The model under review builds one solid part; all positions refer to its coordinate system, in mm. Face numbers are marked on the shaded views. A direction names the side the tool comes from. Coordinates: 2 decimals unless noted, no trailing zeros. Loops run counter-clockwise (first coordinate to the right, second up) from the corner with the lowest first, then second, coordinate; pieces in that order, holes last. Notation, with made-up numbers: M -29,0 L 5,0 A20 cw 5,39 Z; hole C 86.5,81.5 d3. An arc over 180 degrees is marked long. Use one line per item in the form item = value.
Autodesk Fusion 360 part; units mm, degrees
sketch "Sketch1" plane through (0, 0, 0) normal (0, 1, 0) x (1, 0, 0)
  line L0 (65, -5) -> (65, -14.5431)
  line L1 (14.2436, -31.1356) -> (24.2436, -31.1356)
  line L2 (24.2436, -101.1356) -> (14.2436, -101.1356)
  line L3 (14.2436, -101.1356) -> (14.2436, -31.1356)
  line L4 (24.2436, -31.1356) -> (74.2436, -31.1356)
  line L5 (74.2436, -31.1356) -> (74.2436, -41.1356)
  line L6 (74.2436, -41.1356) -> (24.2436, -41.1356)
  line L7 (24.2436, -41.1356) -> (24.2436, -101.1356)
  dimension "d5" = 10
  dimension "d6" = 70
  dimension "d7" = 50
  dimension "d8" = 10
extrude "Extrude1" add sketch "Sketch1" along normal blind 30
sketch "Sketch2" plane through (0, 0, 0) normal (0, 0, 1) x (1, 0, 0)
  circle A0 centre (36, 20) radius 2
  dimension "d11" = 4
extrude "Extrude2" cut sketch "Sketch2" along normal blind 72
pattern_linear "R-Pattern1" count 3 spacing 13 along (1, 0, 0) count 2 spacing 11 along (0, -1, 0) of "Extrude2"
sketch "Sketch3" plane through (0, 0, 0) normal (1, 0, 0) x (0, 0, -1)
  circle A0 centre (-58.7967, 22.3764) radius 2
  dimension "d18" = 4
extrude "Extrude3" cut sketch "Sketch3" along normal blind 50
pattern_linear "R-Pattern2" count 3 spacing 15 along (0, 0, 1) count 2 spacing 15 along (0, -1, 0) of "Extrude3"
fillet "Fillet1" radius 0.5 6 edges at (49.2436, 30, 41.1356) (74.2436, 15, 41.1356) (24.2436, 30, 71.1356) (24.2436, 15, 101.1356) (24.2436, 0, 71.1356) (49.2436, 0, 41.1356)
chamfer "Chamfer1" distance 1 angle 45 12 edges at (34.1353, 9.7232, 41.1356) (47.1353, 9.7232, 41.1356) (60.1353, 9.7232, 41.1356) (60.1353, 20.7232, 41.1356) (47.1353, 20.7232, 41.1356) (34.1353, 20.7232, 41.1356) (24.2436, 8.0997, 60.6613) (24.2436, 8.0997, 75.6613) (24.2436, 8.0997, 90.6613) (24.2436, 23.0997, 75.6613) (24.2436, 23.0997, 90.6613) (24.2436, 23.0997, 60.6613)
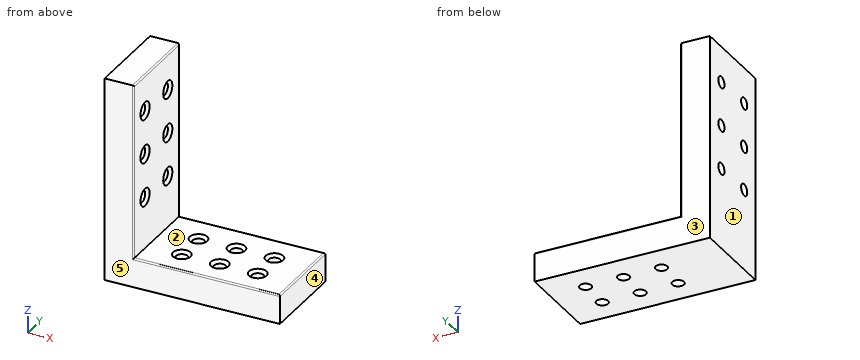
1. Add section A-A (x = 62). State the section outline as (y, z) points.
Response values:
outline = M 0,31.14 L 7,31.14 L 7,40.14 L 6,41.14 L 0.5,41.14 A0.5 ccw 0,40.64 Z; M 11,31.14 L 18,31.14 L 18,40.14 L 17,41.14 L 12,41.14 L 11,40.14 Z; M 22,31.14 L 30,31.14 L 30,40.64 A0.5 ccw 29.5,41.14 L 23,41.14 L 22,40.14 Z
2. Insertion check: P1, Ø1.5, axis at y = 20.5, z = 84, coming from the +X side; P2, Ø3, axis at x = 57, y = 7, coming from the +Z side; P3, Ø4.5, axis at x = 49, y = 9, coming from the +Z side; P4, Ø3, axis at x = 62, y = 9, coming from the +Z side. Each pin has a flat end and moves straight along its axis. Give the tip position at first contact, or say it passes through.
Response values:
P1 = 24.24
P2 = 41.14
P3 = 40.39
P4 = through
3. Wall thickness on line 1 along Y through (x, z) = (36, 37); line 2 along X through (y, z) = (9, 33); line 3 along X through (y, z) = (2, 72): over which ranges is each line inside the solid? List them lowest first. Write a range as from..to.
Response values:
line_1 = 0..7, 11..18, 22..30
line_2 = 14.24..34, 38..47, 51..60, 64..74.24
line_3 = 14.24..24.24
4. Add section C-C (y = 3). State the section outline as (x, z) points.
Response values:
outline = M 14.24,31.14 L 74.24,31.14 L 74.24,40.64 A0.5 ccw 73.74,41.14 L 24.24,41.14 L 24.24,100.64 A0.5 ccw 23.74,101.14 L 14.24,101.14 Z
5. Add section D-D (z = 68). State the section outline as (x, y) points.
Response values:
outline = M 14.24,0 L 23.74,0 A0.5 ccw 24.24,0.5 L 24.24,29.5 A0.5 ccw 23.74,30 L 14.24,30 Z
6. Machinability: for the marked faces 1 and 2, which of the approach directions +Z, -Z, +X, -X, +Y, -Y give a long, thin tool a straight path to every point of the face, cutting with its end or side? Answer none if there is none.
Response values:
face_1 = +Z, -Z, -X, +Y, -Y
face_2 = +Z, +X, +Y, -Y
7. Add section B-B (x = 20.5). State the section outline as (y, z) points, then the cut area to 3 significant figures.
Response values:
outline = M 0,31.14 L 30,31.14 L 30,101.14 L 0,101.14 Z; hole C 7.38,58.8 d4; hole C 7.38,73.8 d4; hole C 7.38,88.8 d4; hole C 22.38,58.8 d4; hole C 22.38,73.8 d4; hole C 22.38,88.8 d4
area = 2,020 mm^2
8. The part is to be moulded in two halves that separate along Y. For the marked faces 3, 4 and 5, say which applies: pulls with the +Y half, pulls with the -Y half, needs draft (parallel to the pull), parting line crosses it, or undercut.
Response values:
face_3 = pulls with the +Y half
face_4 = needs draft
face_5 = pulls with the -Y half
